Could you check a few things on this model? Use its own coordinates, in mm. Give positions to 0.01 mm unless a question says otherwise; leave off trailing zeros. Loops run counter-clockwise (first coordinate to the right, second up) from the corner with the lowest first, then second, coordinate; pieces in that order, holes last. Notation, with made-up numbers: M 55,-15.5 L 109,-15.5 A26 cw 109,13.5 Z; hole C 47,56 d1. An arc over 180 degrees is marked long. Use a Markdown table: item, result. Add a question column.
1) If I drill on line 1 along X through (y, z) = (1.5, 0.45); line 2 along X through (y, z) = (-13.25, 0.4); line 3 along Y through (x, z) = (-16.5, 1.95), over which ranges is the centre line in solid material (lowest first)? Write a range as [from, to].
2) Suppose I cut it at D-D on x = -6.75. List the corners of the cut face in (y, z) for me (3 decimals), and give its area (3 significant figures).
3) Suppose I cut it at C-C on y = -4.25. List the corners of the cut face in (x, z) for me (3 decimals).
4) We'd pull the mould along X, two halves only. Please class faces 1 (the flat face through (0.54, -8.15, 1.57)), 2 (the cylindrical face through (-1.11, -13.98, 1.57)), 3 (the cylindrical face through (-0.31, 1.39, 1.57)): +X half, -X half, draft (parallel to the pull), parting line (faces both ways), or undercut.
5) Suppose I cut it at A-A on z = 1.1. Count the separate pieces of the cut face and the enclosed holes in it, and give its area (3 significant figures).
6) Suppose I cut it at B-B on x = -2.75. List the corners of the cut face in (y, z) for me (3 decimals), and give its area (3 significant figures).
7) Will these pins go through, and if not, where does the flat tip stop? pin 1 Ø1.5 at (y, z) = (-10.5, 3) entering from -X (3 decimals); pin 2 Ø5 at (x, y) = (-7.5, -9.5) entering from -Z.
Autodesk Inventor part; units mm, degrees
ref_plane "YZ Plane" through (0, 0, 0) normal (1, 0, 0) x (0, 1, 0)
ref_plane "XZ Plane" through (0, 0, 0) normal (0, 1, 0) x (-1, 0, 0)
ref_plane "XY Plane" through (0, 0, 0) normal (0, 0, 1) x (1, 0, 0)
sketch "Sketch1" plane through (0, 0, 0) normal (0, 0, 1) x (1, 0, 0)
  circle A0 centre (0, 0) radius 1.4224
  circle A1 centre (0, 0) radius 3.175
  line L0 (0, 0) -> (-15.875, 0) construction
  circle A2 centre (-2.0016, -10.9307) radius 3.175
  circle A3 centre (-2.0016, -10.9307) radius 5 construction
  circle A4 centre (-2.0016, -10.9307) radius 1.5
  line L1 (0, 0) -> (-2.0016, -10.9307) construction
  line L2 (-2.0016, -10.9307) -> (-3.4771, -10.6606) construction
  line L3 (0, 0) -> (-2.0016, -10.9307) construction
  arc A5 (-5.0684, -10.109) -> (1.0652, -11.7525) centre (-2.0016, -10.9307) ccw
  arc A6 (-1.2212, -2.9308) -> (-15.875, 0) centre (-15.875, -38.1) ccw
  arc A7 (-15.875, 3.175) -> (-15.875, 0) centre (-15.875, 1.5875) ccw
  line L4 (-15.875, 3.175) -> (0, 3.175)
  line L5 (-2.0016, -10.9307) -> (-4.9305, 0) construction
  line L6 (1.0652, -10.109) -> (-1.8637, 0.8218)
  line L7 (-7.9973, -0.8218) -> (-5.0684, -11.7525)
  arc A8 (-5.0684, -11.7525) -> (1.0652, -10.109) centre (-2.0016, -10.9307) ccw
  arc A9 (-1.8637, 0.8218) -> (-7.9973, -0.8218) centre (-4.9305, 0) ccw
  circle A10 centre (6.7469, -0.7937) radius 3.175
  circle A11 centre (6.7469, -0.7937) radius 1.5
  line L8 (7.1178, 2.3595) -> (0.371, 3.1533)
  arc A12 (4.6726, -3.1975) -> (-0.0011, -6.1296) centre (2.7869, -5.3826) ccw
  circle A13 centre (6.7469, -0.7937) radius 5 construction
  point P0 (-5.0684, -10.109)
  point P1 (0, 3.175)
  point P2 (-7.9969, -0.8234)
  point P3 (1.0652, -10.109)
  point P4 (-0.8218, -3.0668)
  point P5 (-2.4653, 2.0008)
  point P6 (0.6312, -3.1116)
  point P7 (1.4598, -2.8195)
  point P8 (-1.4243, -1.0642)
  point P9 (-1.7024, 0.5129)
  point P10 (1.0652, -10.109)
  point P11 (-5.0684, -11.7525)
  dimension "d24" = 3
  dimension "d0" = 2.8448
  dimension "d1" = 6.35
  dimension "d9" = 15.875
  dimension "d22" = 6.35
  dimension "d23" = 10
  dimension "d26" = 11.1125
  dimension "d29" = 3.175
  dimension "d30" = 6.35
  dimension "d31" = 6.35
  dimension "d32" = 3
  dimension "d36" = 10
  dimension "d37" = 105
  dimension "d38" = 4.7625
  dimension "d39" = 6.7469
  dimension "d40" = 0.7937
extrude "Extrusion1" add sketch "Sketch1" along normal blind 3.175 contours A1 L6 A9 | A12 L6 A1 | A1 A9 L4 | L6 A2 L7 A6 A1 | A1 A9 L6 | A1 A6 A9 | A9 A6 A7 L4 | A2
fillet "Fillet1" radius 3.175 1 edges at (-7.9969, -0.8234, 1.5875)
properties part number "Lever" material "Aluminum 6061"
Answer block:
| question | item | result |
|---|---|---|
| 1 | line 1 | x = [-17.46, 2.8] |
| 1 | line 2 | x = [-4.17, 0.17] |
| 1 | line 3 | y = [0.13, 3.05] |
| 2 | outline | M -5.477,0 L 3.175,0 L 3.175,3.175 L -5.477,3.175 Z |
| 2 | area | 27.5 mm^2 |
| 3 | outline | M -7.079,0 L 0.132,0 L 0.132,3.175 L -7.079,3.175 Z |
| 4 | face 1 | +X half |
| 4 | face 2 | parting line |
| 4 | face 3 | undercut |
| 5 | separate pieces | 1 |
| 5 | enclosed holes | 2 |
| 5 | area | 153 mm^2 |
| 6 | outline | M -14.016,0 L -12.231,0 L -12.231,3.175 L -14.016,3.175 Z; M -9.631,0 L 3.175,0 L 3.175,3.175 L -9.631,3.175 Z |
| 6 | area | 46.3 mm^2 |
| 7 | pin 1 | stops at x = -5.605 |
| 7 | pin 2 | stops at z = 0 |
